Autodesk Inventor part; units mm, degrees
ref_plane "Work Plane1" through (66.6877, 0, 0) normal (0, 0, -1) x (1, 0, 0)
ref_plane "YZ Plane" through (0, 0, 0) normal (1, 0, 0) x (0, 1, 0)
ref_plane "XZ Plane" through (0, 0, 0) normal (0, 1, 0) x (-1, 0, 0)
sketch "Sketch1" plane through (0, 0, 0) normal (0, 0, 1) x (1, 0, 0)
  line L0 (12.7, 0) -> (12.7, 1.4224)
  line L1 (12.7, 1.4224) -> (2.1082, 1.4224)
  line L2 (0, 2.7686) -> (0, 0.9144)
  line L3 (0, 0.9144) -> (1.397, 0.9144)
  line L4 (1.397, 0.9144) -> (1.9249, 0)
  line L5 (1.9249, 0) -> (12.7, 0)
  line L6 (0, 2.7686) -> (0.5596, 2.7686)
  line L7 (0.5596, 2.7686) -> (2.1082, 1.4224)
  line L8 (-2.54, 0) -> (15.24, 0)
  line L9 (0, -0.5537) -> (0, 3.3223)
  dimension "d0" = 12.7
  dimension "d1" = 1.397
  dimension "d2" = 2.8448
  dimension "d3" = 2.1082
  dimension "d4" = 41
  dimension "d5" = 1.8288
  dimension "d6" = 60
  dimension "d7" = 5.5372
revolve "Body" add sketch "Sketch1" angle 360 about axis through (1.9249, 0, 0) along (1, 0, 0) contours L5 L4 L3 L2 L6 L7 L1 L0
sketch "Sketch2" plane through (0, 0, 0) normal (-1, 0, 0) x (0, 0, 1)
  circle A0 centre (0, 0) radius 2.7686
  circle A1 centre (0, 0) radius 0.9144
  line L0 (0.7066, 0.1893) -> (0.8832, 0.2367)
  line L1 (0.7066, -0.1893) -> (0.8832, -0.2367)
  arc A2 (0.7066, -0.1893) -> (0.7066, 0.1893) centre (0, 0) ccw
  arc A3 (0.8832, -0.2367) -> (0.8832, 0.2367) centre (0, 0) ccw
  line L2 (0, -3.876) -> (0, 3.876)
  line L3 (-3.876, 0) -> (3.876, 0)
  line L4 (0.7066, 0.1893) -> (0, 0) construction
  line L5 (0, 0) -> (0.7066, -0.1893) construction
  line L6 (0.1893, 0.7066) -> (0.2367, 0.8832)
  line L7 (0.5173, 0.5173) -> (0.6466, 0.6466)
  arc A4 (0.5173, 0.5173) -> (0.1893, 0.7066) centre (0, 0) ccw
  arc A5 (0.6466, 0.6466) -> (0.2367, 0.8832) centre (0, 0) ccw
  line L8 (-0.5173, 0.5173) -> (-0.6466, 0.6466)
  line L9 (-0.1893, 0.7066) -> (-0.2367, 0.8832)
  arc A6 (-0.1893, 0.7066) -> (-0.5173, 0.5173) centre (0, 0) ccw
  arc A7 (-0.2367, 0.8832) -> (-0.6466, 0.6466) centre (0, 0) ccw
  line L10 (-0.7066, -0.1893) -> (-0.8832, -0.2367)
  line L11 (-0.7066, 0.1893) -> (-0.8832, 0.2367)
  arc A8 (-0.7066, 0.1893) -> (-0.7066, -0.1893) centre (0, 0) ccw
  arc A9 (-0.8832, 0.2367) -> (-0.8832, -0.2367) centre (0, 0) ccw
  line L12 (-0.1893, -0.7066) -> (-0.2367, -0.8832)
  line L13 (-0.5173, -0.5173) -> (-0.6466, -0.6466)
  arc A10 (-0.5173, -0.5173) -> (-0.1893, -0.7066) centre (0, 0) ccw
  arc A11 (-0.6466, -0.6466) -> (-0.2367, -0.8832) centre (0, 0) ccw
  line L14 (0.5173, -0.5173) -> (0.6466, -0.6466)
  line L15 (0.1893, -0.7066) -> (0.2367, -0.8832)
  arc A12 (0.1893, -0.7066) -> (0.5173, -0.5173) centre (0, 0) ccw
  arc A13 (0.2367, -0.8832) -> (0.6466, -0.6466) centre (0, 0) ccw
  dimension "d8" = 1.463
  dimension "d9" = 1.8288
  dimension "d10" = 15
  dimension "d11" = 15
  dimension "d22" = 360
extrude "Slot" add sketch "Sketch2" against normal up to next contours L3 A2 L0 A1 | A1 L1 A2 L3 | L3 A8 L10 A1 | A1 L11 A8 L3 | A1 L7 A4 L6 | L9 A6 L8 A1 | A1 L13 A10 L12 | L15 A12 L14 A1
thread "Thread"
chamfer "Chamfer1" distance 0.3785 distance2 0.7569 1 edges at (12.7, -1.4224, 0) measured on face at (12.7, -0.1681, 0.4433)
ref_plane "Work Plane1" through (66.6877, 0, 0) normal (0, 0, -1) x (1, 0, 0)
equation "\"d0\" = NLG"
equation "\"d1\" = INTI"
equation "\"d2\" = GD"
equation "\"d3\" = KOH"
equation "\"d4\" = 0.5 * SEWI"
equation "\"d5\" = SW"
equation "\"d7\" = KOD"
equation "\"d8\" = 0.8 * SW"
equation "\"d9\" = SW"
equation "\"d15\" = GEL"
equation "\"d17\" = -0.5 * SPD + 0.5 * GD"
equation "\"d18\" = GUL"
equation "\"NLG\" = 12.7"
equation "\"SW\" = 1.8288"
equation "\"INTI\" = 1.397"
equation "\"GEL\" = 9.0043"
equation "\"KOH\" = 2.1082"
equation "\"KOD\" = 5.5372"
equation "\"GUL\" = 0.75692"
equation "\"SPD\" = 2.08788"
equation "\"GD\" = NND"
equation "\"SEWI\" = 82deg"
equation "\"TOA\" = 30deg"
equation "\"GD1\" = SPD"
equation "\"EPV\" = 3.74448"
equation "\"THREADDIA\" = 2.8448"
equation "\"BDM\" = NND"
equation "\"NND\" = 2.8448"
equation "\"GAL\" = 1.5875"
equation "\"E0\" = 1.155 * SW"
properties part number "ANSI B18.3 - 4-40 UNC x 0.5, SSFCHCSI" material "Steel, Mild"
The model under review builds one solid part; all positions refer to its coordinate system, in mm. Coordinates: 2 decimals unless noted, no trailing zeros. Loops run counter-clockwise (first coordinate to the right, second up) from the corner with the lowest first, then second, coordinate; pieces in that order, holes last.
(1) Consider section A-A, the plane x = 10.25. Give the boundary of the cut face in (y, z), plus the area to 3 significant figures.
Determined:
outline: circle Ø2.84 at (0, 0)
area: 6.36 mm2
(2) Wall thickness on L1, parallel to Y at x = 6.25, z = 0.05; L2, parallel to Y at x = 11.5, z = -0.7: over which ranges is each line inside the solid? List them lowest first.
Determined:
L1: y = -1.42 to 1.42
L2: y = -1.24 to 1.24
(3) Draft analysis for pull direction Z (two halves, no side actions). For faces 1 (the flat face through (12.7, 0, 0)), 2 (the cylindrical face through (6.96, -0.31, 1.39)), 3 (the conical face through (1.89, 0.03, -0.05)), state which applies: +Z half, -Z half, draft (parallel to the pull), parting line (faces both ways), or undercut.
Determined:
face 1: draft
face 2: parting line
face 3: undercut
(4) Insertion check: P1, Ø1.5, axis at x = 3.5, z = 0.5, coming from the +Y side. The pin has a flat end and moves straight along its axis. Give the tip position at first contact, or say it passes through.
Determined:
P1: stops at y = 1.42
